Part model, mm, in its own coordinate system. Face numbers are marked on the shaded views. Give positions to 0.01 mm unless a question says otherwise; leave off trailing zeros. Order: outer loops, then holes, each group sorted by start corner. A loop starts at its lowest first (then second) coordinate and runs counter-clockwise, first axis right, second up. Notation, with made-up numbers: M 50.5,65 L 85.5,65 A23 cw 85.5,83 Z; hole C 19,-30.75 d1. An arc over 180 degrees is marked long. Answer as a JSON object with one key per item and string values.
from build123d import *

# Parameters (mm, degrees)
BEARING_DIMENSIONS_R   = 21
BEARING_DIMENSIONS_R_2 = 10
BEARING_EXTRUDE_DEPTH  = 6
FILLET1_R              = 1


with BuildPart() as part:
    # Bearing Dimensions → Bearing Extrude (new, symmetric)
    with BuildSketch(Plane.XY):
        Circle(BEARING_DIMENSIONS_R)
        Circle(BEARING_DIMENSIONS_R_2, mode=Mode.SUBTRACT)
    extrude(amount=BEARING_EXTRUDE_DEPTH, both=True)

    # Fillet1
    fillet1_edges = [part.edges().sort_by_distance(p)[0] for p in [
        (-21, 0, -6),
        (-21, 0, 6),
        (-10, 0, -6),
        (-10, 0, 6),
    ]]
    fillet(fillet1_edges, radius=FILLET1_R)


solid = part.part
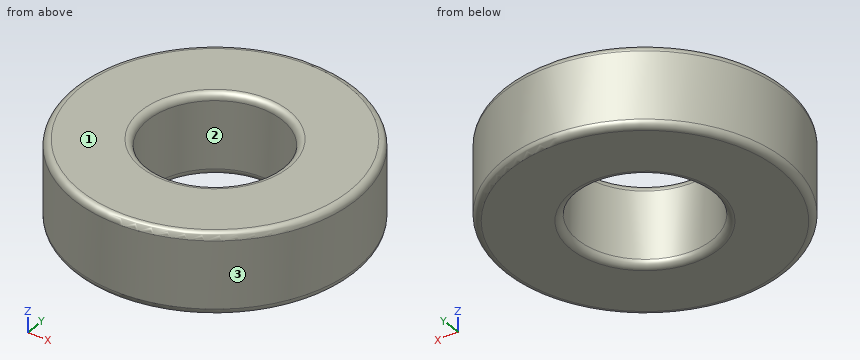
1. Two-plate mould, pull along Y, no slides. Class the marked faces 1, 2 and 3: +Y half, -Y half, draft (parallel to the pull), parting line (faces both ways), or undercut.
Worked answers:
{"face 1": "draft", "face 2": "undercut", "face 3": "parting line"}
2. Pin check, flat tips, straight feed: P1, Ø5, axis at x = 13, z = 3, coming from the -Y side; P2, Ø2, axis at y = -14.5, z = 3.5, coming from the +X side; P3, Ø12, axis at x = 0, y = 0, coming from the +Z side; P4, Ø2, axis at y = 15, z = -4, coming from the -X side. Stop position of each tip, or through.
Worked answers:
{"P1": "stops at y = -18.19", "P2": "stops at x = 16.09", "P3": "passes through", "P4": "stops at x = -15.65"}
3. Cut at A-A on x = 0. Give the cut face in (y, z).
Worked answers:
{"outline": "M -21,-5 A1 ccw -20,-6 L -11,-6 A1 ccw -10,-5 L -10,5 A1 ccw -11,6 L -20,6 A1 ccw -21,5 Z; M 10,-5 A1 ccw 11,-6 L 20,-6 A1 ccw 21,-5 L 21,5 A1 ccw 20,6 L 11,6 A1 ccw 10,5 Z"}
4. Cut at C-C on z = 0. Give the cut face in (x, y), plus the area to 3 significant figures.
Worked answers:
{"outline": "C 0,0 d42; hole C 0,0 d20", "area": "1,070 mm^2"}
5. Probe line 1 along Y through (x, z) = (0, 0.5); line 2 along X through (y, z) = (6, 1.5); line 3 along X through (y, z) = (-4, -3). List the from-to ranges inside material, lowest first.
Worked answers:
{"line 1": "y = -21 to -10, 10 to 21", "line 2": "x = -20.12 to -8, 8 to 20.12", "line 3": "x = -20.62 to -9.17, 9.17 to 20.62"}
